Check sheet for the modelled part. Datum: model origin and axes. Units: mm. A direction names the side the tool comes from. Coordinates: 2 decimals unless noted, no trailing zeros. Loops run counter-clockwise (first coordinate to the right, second up) from the corner with the lowest first, then second, coordinate; pieces in that order, holes last. Notation, with made-up numbers: (23.25, 38) - (55.25, 38) arc R26 cw to (55.25, 54) - close; hole circle Ø4 at (44.5, 28). An arc over 180 degrees is marked (long way). Use a Markdown table: item, result. Add a question column.
1) Draft check along X on faces 4 (the flat face through (-12.135, -3.5, -0.5)), 5 (the flat face through (9, 3.5, 4.4)), 6 (the flat face through (10, 4, 3)). Enter one of: pulls with the +X half, pulls with the -X half, needs draft (parallel to the pull), parting line crosses it, or undercut.
2) Go/stop test with flat-tipped pins: P1, Ø1.1, axis at x = 3.5, z = 4, coming from the +Y side; P2, Ø13, axis at x = 0, y = 0, coming from the -Z side; P3, Ø3.5, axis at y = -10.5, z = 4.5, coming from the -X side. Record where each tip stops, or that it passes through.
3) Sectioned sample at B-B, the plane z = 5.5. Enter the section's corners in (x, y), then the cut area to 3 significant figures.
4) Thickness scan on line 1 (Y direction, x = 0, z = 8.75); line 2 (Z direction, x = 10.5, y = 0.5); line 3 (X direction, y = 1.5, z = -0.5). Record the ranges inside material, lowest first.
5) Tool access check on faces 1 (the flat face through (-10, -3, 4)), 2 (the flat face through (3, -10, 4)), 3 (the flat face through (-3.5, 9, 4.4)). Record the directions out of +Z, -Z, +X, -X, +Y, -Y that give a thin tool (end or side, any length) a straight path to the whole face; none if there is none.
6) Sectioned sample at D-D, the plane z = 7.5. Enter the section's corners in (x, y), then the cut area to 3 significant figures.
7) Sectioned sample at A-A, the plane y = 0. Enter the section's corners in (x, z).
from build123d import *

# Parameters (mm, degrees)
CUT_EXTRUDE1_REACH  = 22.821
SKETCH2_W           = 5.674675786
SKETCH2_H           = 3.1346611
BOSS_EXTRUDE1_DEPTH = 1
CIRPATTERN1_COUNT   = 4


with BuildPart() as part:
    # Sketch1 → Revolve-Thin2 (revolve)
    with BuildSketch(Plane.YZ, mode=Mode.PRIVATE) as revolve_thin2_sk:
        with BuildLine():
            Line((5, 11), (5, 2))
            ThreePointArc((5, 2), (5.585786438, 0.585786438), (7, 0))
            Line((7, 0), (12.5, 0))
            Line((12.5, 0), (12.5, -1))
            Line((12.5, -1), (7, -1))
            ThreePointArc((7, -1), (4.878679656, -0.121320344), (4, 2))
            Line((4, 2), (4, 11))
            Line((4, 11), (5, 11))
        make_face()
    revolve(revolve_thin2_sk.sketch.rotate(Axis((0, 0, 14.992157351), (0, 0, -1)), 90), axis=Axis((0, 0, 14.992157351), (0, 0, -1)))

    # Sketch2 → Cut-Extrude1 (cut, up to next)
    with BuildSketch(Plane(origin=(0, 0, 0), x_dir=(0, 1, 0), z_dir=(0, 0, 1)), mode=Mode.PRIVATE) as cut_extrude1_sk1:
        with Locations((-5.837337893, 10.56733055)):
            Rectangle(SKETCH2_W, SKETCH2_H)
    cut_extrude1_tool1 = extrude(cut_extrude1_sk1.sketch, amount=-CUT_EXTRUDE1_REACH, mode=Mode.PRIVATE) & part.part
    cut_extrude1 = cut_extrude1_tool1.solids().sort_by_distance((-10.567331, -5.837338, 0))[0]
    add(cut_extrude1, mode=Mode.SUBTRACT)

    # Sketch3 → Boss-Extrude1 (add)
    with BuildSketch(Plane.XZ.offset(3)):
        with BuildLine():
            Line((-9, -1), (-9, 9))
            ThreePointArc((-9, 9), (-11.328570013, 4.765136415), (-12.1346611, 0))
            Line((-12.1346611, 0), (-12.1346611, -1))
            Line((-12.1346611, -1), (-9, -1))
        make_face()
    boss_extrude1 = extrude(amount=BOSS_EXTRUDE1_DEPTH)

    # CirPattern1: Cut-Extrude1, Boss-Extrude1 ×4 about axis
    cirpattern1_axis = Axis((0, 0, 0), (0, 0, 1))
    add([cut_extrude1.rotate(cirpattern1_axis, i * 360 / CIRPATTERN1_COUNT) for i in range(1, CIRPATTERN1_COUNT)], mode=Mode.SUBTRACT)
    add([boss_extrude1.rotate(cirpattern1_axis, i * 360 / CIRPATTERN1_COUNT) for i in range(1, CIRPATTERN1_COUNT)])


solid = part.part
Solved:
| question | item | result |
|---|---|---|
| 1 | face 4 | pulls with the -X half |
| 1 | face 5 | undercut |
| 1 | face 6 | needs draft |
| 2 | P1 | stops at y = 4.04 |
| 2 | P2 | stops at z = -0.96 |
| 2 | P3 | stops at x = 3 |
| 3 | outline | (-11.05, -4) - (-9, -4) - (-9, -3) - (-11.05, -3) - close; circle Ø10 at (0, 0); (-4, 9) - (-3, 9) - (-3, 11.05) - (-4, 11.05) - close; (3, -11.05) - (4, -11.05) - (4, -9) - (3, -9) - close; (9, 3) - (11.05, 3) - (11.05, 4) - (9, 4) - close; hole circle Ø8 at (0, 0) |
| 3 | area | 36.5 mm2 |
| 4 | line 1 | y = -5 to -4, 4 to 5 |
| 4 | line 2 | z = -1 to 0 |
| 4 | line 3 | x = -12.41 to -5.13, 5.13 to 12.41 |
| 5 | face 1 | +Z, -X, +Y |
| 5 | face 2 | +Z, -X, -Y |
| 5 | face 3 | +Z, +X, -X |
| 6 | outline | (-10.04, -4) - (-9, -4) - (-9, -3) - (-10.04, -3) - close; circle Ø10 at (0, 0); (-4, 9) - (-3, 9) - (-3, 10.04) - (-4, 10.04) - close; (3, -10.04) - (4, -10.04) - (4, -9) - (3, -9) - close; (9, 3) - (10.04, 3) - (10.04, 4) - (9, 4) - close; hole circle Ø8 at (0, 0) |
| 6 | area | 32.4 mm2 |
| 7 | outline | (-12.5, -1) - (-7, -1) arc R3 ccw to (-4, 2) - (-4, 11) - (-5, 11) - (-5, 2) arc R2 cw to (-7, 0) - (-12.5, 0) - close; (4, 2) arc R3 ccw to (7, -1) - (12.5, -1) - (12.5, 0) - (7, 0) arc R2 cw to (5, 2) - (5, 11) - (4, 11) - close |
